The listing builds one solid part. Answer for the finished solid, in the listing's coordinates (mm). Face numbers are marked on the shaded views. Give positions to 0.01 mm unless a question says otherwise; leave off trailing zeros. Write each loop counter-clockwise with the first axis right and the second up, starting at its lowest first coordinate (ties: lowest second). Pieces come first, ordered by that corner, then holes. Notation, with made-up numbers: (-30, 61.25) - (-5, 61.25) arc R20 ccw to (-5, 65.25) - close; hole circle Ø7 at (24.5, -40). An arc over 180 degrees is marked (long way). Answer as CSV lines item,"result". Start each with the question number.
(1) Find section C-C (y = 1.65). Write down the section's boundary in (x, z) (3 decimals), then the cut area to 3 significant figures.
(2) Find section B-B (z = 0). Write down the section's boundary in (x, y) (3 decimals), then the cut area to 4 significant figures.
(3) Straight lines are drawn through the part: probe 1 along Z at (x, y) = (0, 1.05) (3 decimals); probe 2 along Z at (x, y) = (0.85, 1.35) (3 decimals); probe 3 along X at (y, z) = (1.8, -0.45) (3 decimals). For each, find the intervals that lie inside material, in ascending order.
(4) For a pull along X with two mould halves and no side action, classify the marked faces 1, 2, 3 and 4 as pulls with the +X half, pulls with the -X half, needs draft (parallel to the pull), parting line crosses it, or undercut.
(5) Find section A-A (x = 0). Write down the section's boundary in (y, z) (3 decimals).
Autodesk Inventor part; units mm, degrees
ref_plane "YZ Plane" through (0, 0, 0) normal (1, 0, 0) x (0, 1, 0)
ref_plane "XZ Plane" through (0, 0, 0) normal (0, 1, 0) x (-1, 0, 0)
ref_plane "XY Plane" through (0, 0, 0) normal (0, 0, 1) x (1, 0, 0)
sketch "Sketch1" plane through (0, 0, 0) normal (0, 1, 0) x (-1, 0, 0)
  line L0 (-2.925, 2.925) -> (2.925, 2.925)
  line L1 (2.925, 2.925) -> (2.925, -2.925)
  line L2 (2.925, -2.925) -> (-2.925, -2.925)
  line L3 (-2.925, -2.925) -> (-2.925, 2.925)
  circle A0 centre (0, 0) radius 1.675
  point P0 (0, 2.925)
  point P1 (2.925, 0)
  dimension "d0" = 5.85
  dimension "d1" = 3.35
extrude "Extrusion1" add sketch "Sketch1" along normal blind 2.15
equation "\"d0\" = nut_A"
equation "\"d1\" = nut_C"
equation "\"d2\" = nut_B"
properties part number "NUT_3MM"
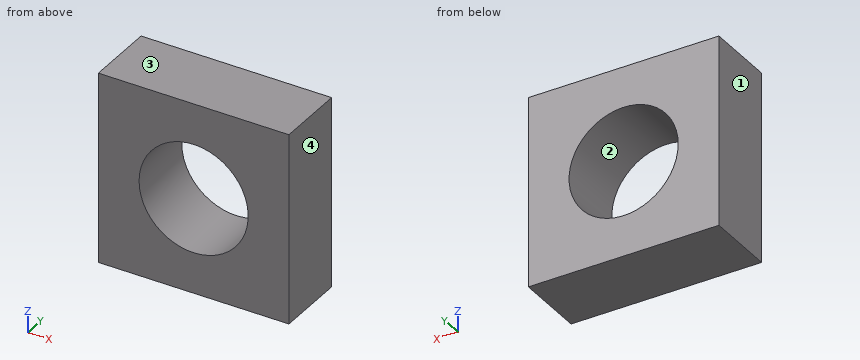
Result set:
1,outline,"(-2.925, -2.925) - (2.925, -2.925) - (2.925, 2.925) - (-2.925, 2.925) - close; hole circle Ø3.35 at (0, 0)"
1,area,"25.4 mm^2"
2,outline,"(-2.925, 0) - (-1.675, 0) - (-1.675, 2.15) - (-2.925, 2.15) - close; (1.675, 0) - (2.925, 0) - (2.925, 2.15) - (1.675, 2.15) - close"
2,area,"5.375 mm^2"
3,probe 1,"-2.925 to -1.675, 1.675 to 2.925"
3,probe 2,"-2.925 to -1.443, 1.443 to 2.925"
3,probe 3,"-2.925 to -1.613, 1.613 to 2.925"
4,face 1,"pulls with the -X half"
4,face 2,"undercut"
4,face 3,"needs draft"
4,face 4,"pulls with the +X half"
5,outline,"(0, -2.925) - (2.15, -2.925) - (2.15, -1.675) - (0, -1.675) - close; (0, 1.675) - (2.15, 1.675) - (2.15, 2.925) - (0, 2.925) - close"
